Check sheet for the modelled part. Datum: model origin and axes. Units: mm. Face numbers are marked on the shaded views. A direction names the side the tool comes from. Coordinates: 2 decimals unless noted, no trailing zeros. Loops run counter-clockwise (first coordinate to the right, second up) from the corner with the lowest first, then second, coordinate; pieces in that order, holes last.
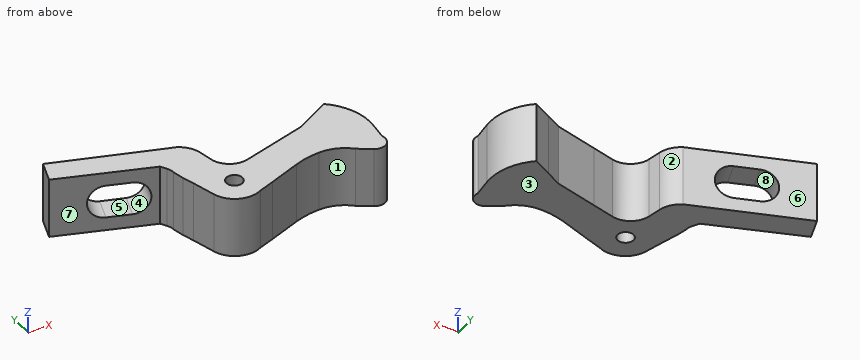
```python
from build123d import *

# Parameters (mm, degrees)
ESQUISSE1_R             = 2.420540081
BOSS_EXTRU_1_DEPTH      = 18
ENL_V_MAT_EXTRU_1_DEPTH = 39.789502353


with BuildPart() as part:
    # Esquisse1 → Boss.-Extru.1 (new body)
    with BuildSketch(Plane.XY):
        with BuildLine():
            Line((7.309445695, 53.714347138), (40.857601275, 42.311087759))
            ThreePointArc((40.857601275, 42.311087759), (43.397194427, 40.141751778), (44.749299605, 37.087678504))
            Line((44.749299605, 37.087678504), (45.525391945, 33.121685243))
            ThreePointArc((45.525391945, 33.121685243), (48.466826033, 28.880719759), (53.578886424, 28.170324589))
            Line((53.578886424, 28.170324589), (60.334857797, 30.077073056))
            Line((60.334857797, 30.077073056), (73.18964939, 33.705101183))
            Line((73.18964939, 33.705101183), (77.686625145, 36.255437702))
            Line((77.686625145, 36.255437702), (83.301564432, 39.439796589))
            ThreePointArc((83.301564432, 39.439796589), (88.190630708, 32.808798216), (89.3438897, 24.651402666))
            Line((89.3438897, 24.651402666), (88.758364996, 19.199881093))
            ThreePointArc((88.758364996, 19.199881093), (87.769834705, 15.522983246), (83.96770833, 15.321476572))
            Line((83.96770833, 15.321476572), (79.922264923, 17.941129356))
            ThreePointArc((79.922264923, 17.941129356), (75.820018568, 20.528976888), (71.032935331, 21.309498572))
            ThreePointArc((71.032935331, 21.309498572), (67.034937106, 20.827330487), (63.167207989, 19.706104665))
            Line((63.167207989, 19.706104665), (53.880076109, 16.176154046))
            Line((53.880076109, 16.176154046), (49.199654782, 14.466799098))
            ThreePointArc((49.199654782, 14.466799098), (42.490348453, 14.160285015), (38.050617194, 19.199881093))
            Line((38.050617194, 19.199881093), (36.098238925, 26.117527504))
            Line((36.098238925, 26.117527504), (35.016515722, 29.633127914))
            Line((35.016515722, 29.633127914), (34.2322664, 33.121685243))
            ThreePointArc((34.2322664, 33.121685243), (34.067751372, 34.27153749), (33.610275558, 35.339217809))
            Line((33.610275558, 35.339217809), (32.57129733, 37.087678504))
            Line((32.57129733, 37.087678504), (4.96334494, 46.812166758))
            Line((4.96334494, 46.812166758), (7.309445695, 53.714347138))
        make_face()
        with Locations((45.822816194, 21.878618475)):
            Circle(ESQUISSE1_R, mode=Mode.SUBTRACT)
    extrude(amount=BOSS_EXTRU_1_DEPTH)

    # Esquisse2 → Enlèv. mat.-Extru.1 (cut, through all)
    with BuildSketch(Plane(origin=(17.123954965, 50.378324845, 0), x_dir=(0.946799522, -0.321823967, 0), z_dir=(0.321823967, 0.946799522, 0))):
        with BuildLine():
            Line((4.63401539, -14), (11.63401539, -14))
            ThreePointArc((11.63401539, -14), (16.63401539, -9), (11.63401539, -4))
            Line((11.63401539, -4), (4.63401539, -4))
            ThreePointArc((4.63401539, -4), (-0.36598461, -9), (4.63401539, -14))
        make_face()
    extrude(amount=-ENL_V_MAT_EXTRU_1_DEPTH, mode=Mode.SUBTRACT)


solid = part.part
```
1) Set-up check for the marked faces 1, 2, 3, 4 and 5: record each of +Z, -Z, +X, -X, +Y, -Y from which the full face is reachable in a straight line by a thin tool's end or side.
Answer sheet:
face 1: +Z, -Z, -Y
face 2: +Z, -Z, +Y
face 3: -Z, +X, -X, +Y, -Y
face 4: +Y
face 5: none
2) Section check B-B on z = 15.75. Enter the section's corners in (x, y).
Answer sheet:
outline: (4.96, 46.81) - (32.57, 37.09) - (33.61, 35.34) arc R4.43 cw to (34.23, 33.12) - (35.02, 29.63) - (36.1, 26.12) - (38.05, 19.2) arc R7.77 ccw to (49.2, 14.47) - (53.88, 16.18) - (63.17, 19.71) arc R24.86 cw to (71.03, 21.31) arc R12.17 cw to (79.92, 17.94) - (83.97, 15.32) arc R3.24 ccw to (88.76, 19.2) - (89.34, 24.65) arc R16.82 ccw to (83.3, 39.44) - (73.19, 33.71) - (53.58, 28.17) arc R6.43 cw to (45.53, 33.12) - (44.75, 37.09) arc R7.53 ccw to (40.86, 42.31) - (7.31, 53.71) - close; hole circle Ø4.84 at (45.82, 21.88)
3) Mould release check, pull along X, two halves, no side actions. Record for the marked faces 6, 7 and 8: +X half, -X half, draft (parallel to the pull), parting line (faces both ways), or undercut.
Answer sheet:
face 6: +X half
face 7: -X half
face 8: undercut
4) Section check A-A on z = 9.75. Enter the section's corners in (x, y).
Answer sheet:
outline: (4.96, 46.81) - (14.45, 43.47) - (16.83, 50.48) - (7.31, 53.71) - close; (30.38, 37.86) - (32.57, 37.09) - (33.61, 35.34) arc R4.43 cw to (34.23, 33.12) - (35.02, 29.63) - (36.1, 26.12) - (38.05, 19.2) arc R7.77 ccw to (49.2, 14.47) - (53.88, 16.18) - (63.17, 19.71) arc R24.86 cw to (71.03, 21.31) arc R12.17 cw to (79.92, 17.94) - (83.97, 15.32) arc R3.24 ccw to (88.76, 19.2) - (89.34, 24.65) arc R16.82 ccw to (83.3, 39.44) - (73.19, 33.71) - (53.58, 28.17) arc R6.43 cw to (45.53, 33.12) - (44.75, 37.09) arc R7.53 ccw to (40.86, 42.31) - (32.82, 45.04) - close; hole circle Ø4.84 at (45.82, 21.88)
5) Scan lines: line 1 (Z direction, x = 24, y = 45.5); line 2 (X direction, y = 35, z = 10); line 3 (X direction, y = 39, z = 10.5). Record each from-to range of solid material in increasing order.
Answer sheet:
line 1: z = 0 to 4, 14 to 18
line 2: x = 33.79 to 45.16, 75.47 to 87.1
line 3: x = 30.58 to 44.1, 82.53 to 83.82
6) Section check D-D on x = 69.5. Enter the section's corners in (y, z), plus the area to 3 significant figures.
Answer sheet:
outline: (21.2, 0) - (32.66, 0) - (32.66, 18) - (21.2, 18) - close
area: 206 mm2
7) Depth check by flat-ended pin: pin 1 (1.5 mm diameter, centred on y = 21, z = 3.5, fed in from +X); pin 2 (4 mm diameter, centred on x = 76, z = 12, fed in from +Y); pin 3 (6 mm diameter, centred on y = 45, z = 8, fed in from +X). Enter the tip coordinate at first touch or a pass-through.
Answer sheet:
pin 1: stops at x = 89.03
pin 2: stops at y = 36.43
pin 3: stops at x = 41.4
8) Section check C-C on z = 5.75. Enter the section's corners in (x, y), plus the area to 3 significant figures.
Answer sheet:
outline: (4.96, 46.81) - (15.53, 43.09) - (17.91, 50.11) - (7.31, 53.71) - close; (29.3, 38.24) - (32.57, 37.09) - (33.61, 35.34) arc R4.43 cw to (34.23, 33.12) - (35.02, 29.63) - (36.1, 26.12) - (38.05, 19.2) arc R7.77 ccw to (49.2, 14.47) - (53.88, 16.18) - (63.17, 19.71) arc R24.86 cw to (71.03, 21.31) arc R12.17 cw to (79.92, 17.94) - (83.97, 15.32) arc R3.24 ccw to (88.76, 19.2) - (89.34, 24.65) arc R16.82 ccw to (83.3, 39.44) - (73.19, 33.71) - (53.58, 28.17) arc R6.43 cw to (45.53, 33.12) - (44.75, 37.09) arc R7.53 ccw to (40.86, 42.31) - (31.74, 45.41) - close; hole circle Ø4.84 at (45.82, 21.88)
area: 997 mm2
